```python
from build123d import *

# Parameters (mm, degrees)
ESBO_O1_R                = 2.975
RESSALTO_EXTRUS_O1_DEPTH = 10
ESBO_O2_R                = 4.073112834
ESBO_O2_R_2              = 2.425
CORTE_EXTRUS_O1_DEPTH    = 1.12
ESBO_O3_R                = 1.455
CORTE_EXTRUS_O2_DEPTH    = 1
ESBO_O4_R                = 1.975
CORTE_EXTRUS_O3_DEPTH    = 9
RESSALTO_EXTRUS_O2_START = 0.5
ESBO_O5_R                = 1.975
RESSALTO_EXTRUS_O2_DEPTH = 0.5
CHANFRO1_SIZE            = 0.25
ESBO_O6_W                = 0.8
ESBO_O6_H                = 6.683609012
CORTE_EXTRUS_O4_DEPTH    = 3
CHANFRO2_SIZE            = 0.5
ESBO_O7_W                = 0.7
ESBO_O7_H                = 5.908680056
RESSALTO_EXTRUS_O3_DEPTH = 6


with BuildPart() as part:
    # Esboço1 → Ressalto-extrusão1 (new body)
    with BuildSketch(Plane.XY):
        Circle(ESBO_O1_R)
    extrude(amount=RESSALTO_EXTRUS_O1_DEPTH)

    # Esboço2 → Corte-extrusão1 (cut)
    with BuildSketch(Plane(origin=(0, 0, 5.5), x_dir=(-1, 0, 0), z_dir=(0, 0, -1))):
        Circle(ESBO_O2_R)
        Circle(ESBO_O2_R_2, mode=Mode.SUBTRACT)
    extrude(amount=-CORTE_EXTRUS_O1_DEPTH, mode=Mode.SUBTRACT)

    # Esboço3 → Corte-extrusão2 (cut)
    with BuildSketch(Plane(origin=(0, 0, 0), x_dir=(-1, 0, 0), z_dir=(0, 0, -1))):
        Circle(ESBO_O3_R)
    extrude(amount=-CORTE_EXTRUS_O2_DEPTH, mode=Mode.SUBTRACT)

    # Esboço4 → Corte-extrusão3 (cut)
    with BuildSketch(Plane.XY.offset(10)):
        Circle(ESBO_O4_R)
    extrude(amount=-CORTE_EXTRUS_O3_DEPTH, mode=Mode.SUBTRACT)

    # Esboço5 → Ressalto-extrusão2 (add)
    with BuildSketch(Plane.XY.offset(1).offset(RESSALTO_EXTRUS_O2_START)):
        Circle(ESBO_O5_R)
    extrude(amount=-RESSALTO_EXTRUS_O2_DEPTH)

    # Chanfro1
    chanfro1_edges = [part.edges().sort_by_distance(p)[0] for p in [
        (-2.975, 0, 0),
        (-2.975, 0, 10),
    ]]
    chamfer(chanfro1_edges, length=CHANFRO1_SIZE)

    # Esboço6 → Corte-extrusão4 (cut)
    with BuildSketch(Plane.XY.offset(10)):
        Rectangle(ESBO_O6_W, ESBO_O6_H)
    extrude(amount=-CORTE_EXTRUS_O4_DEPTH, mode=Mode.SUBTRACT)

    # Chanfro2
    # the kernel refuses this chamfer: 0.5 mm, written as the material it takes off along each edge
    with BuildSketch(Plane(origin=(0.4, 0.64822805, 10), x_dir=(-0.027495876610586403, 0, -0.9996219169112968), z_dir=(0, 1, 0))) as chanfro2_piece_1:
        Polygon((CHANFRO2_SIZE * 0.999621916911, -CHANFRO2_SIZE * 0.0274958766106), (-CHANFRO2_SIZE * 0.0274958766106, -CHANFRO2_SIZE * 0.999621916911), (0, 0), align=None)
    extrude(amount=3.333095776, mode=Mode.SUBTRACT)
    with BuildSketch(Plane(origin=(0.4, -3.981323826, 10), x_dir=(0.9996219169112968, 0, 0.027495876610585633), z_dir=(0, 1, 0)), Plane(origin=(-0.4, -0.64822805, 10), x_dir=(-0.9996219169112968, 0, 0.027495876610585623), z_dir=(0, -1, 0)), Plane(origin=(-0.4, 3.981323826, 10), x_dir=(-0.9996219169112968, 0, 0.027495876610585623), z_dir=(0, -1, 0))) as chanfro2_piece_2:
        Polygon((CHANFRO2_SIZE * 0.999621916911, CHANFRO2_SIZE * 0.0274958766106), (-CHANFRO2_SIZE * 0.0274958766106, CHANFRO2_SIZE * 0.999621916911), (0, 0), align=None)
    extrude(amount=3.333095776, mode=Mode.SUBTRACT)

    # Esboço7 → Ressalto-extrusão3 (add)
    with BuildSketch(Plane.XY.offset(7)):
        Rectangle(ESBO_O7_W, ESBO_O7_H)
    extrude(amount=RESSALTO_EXTRUS_O3_DEPTH)


solid = part.part
```
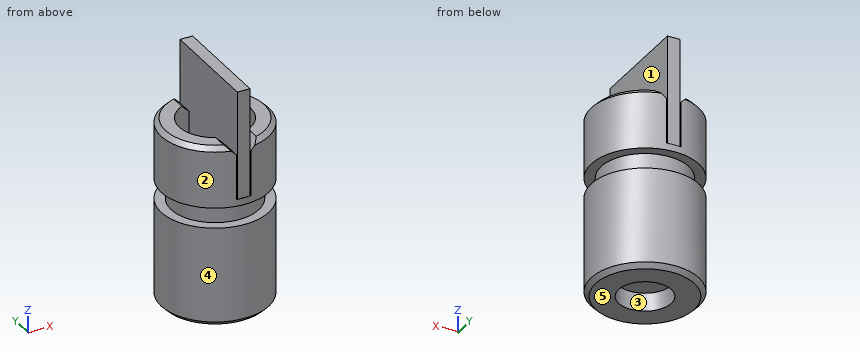
For this review, take the finished solid that the model builds, in its own axes (mm). Face numbers are marked on the shaded views. A direction names the side the tool comes from. Coordinates: 2 decimals unless noted, no trailing zeros. Loops run counter-clockwise (first coordinate to the right, second up) from the corner with the lowest first, then second, coordinate; pieces in that order, holes last. Notation, with made-up numbers: (87, 78.5) - (136, 78.5) arc R17 cw to (136, 103.5) - close; hole circle Ø4 at (-33, 8.25). An arc over 180 degrees is marked (long way). Use one line per item in the form item = value. Start each with the question number.
1) Take a section at B-B (x = 0). State the section outline as (y, z) points (3 decimals).
2) Draft analysis for pull direction X (two halves, no side actions). For the marked faces 3, 4 and 5, state which applies: released by +X, released by -X, zero draft, split by the parting line, or undercut.
3) Take a section at C-C (z = 4.25). State the section outline as (x, y) points (3 decimals), plus the area to 3 significant figures.
4) Take a section at A-A (y = 0). State the section outline as (x, z) points (3 decimals), plus the area to 3 significant figures.
5) For pin 1 (0.6 mm diameter, centred on x = 0, z = 9.5, fed in from +Y); pin 2 (1 mm diameter, centred on x = -0.5, z = 4.5, fed in from -Y) (3 decimals); pin 3 (0.8 mm diameter, centred on y = -2.5, z = 8, fed in from -X); pin 4 (1.5 mm diameter, centred on x = -1.5, y = -0.5, fed in from +Z), all flat-tipped, find the tip position at first contact; note any pin that passes through.
6) For the marked faces 1 and 2, list the 3-axis set-ups (+Z, -Z, +X, -X, +Y, -Y) from which the entire face can be reached by the end or side of a thin tool; tool diameter is ignored.
7) To check wall thickness, follow probe 1 along Z at (x, y) = (0.15, -0.45); probe 2 along Z at (x, y) = (1.2, 2.25); probe 3 along X at (y, z) = (0, 3.5) (3 decimals). State the ranges of each line that lie inside material, in increasing order. Write a range as from..to.
8) Take a section at D-D (z = 11). State the section outline as (x, y) points.
From the geometry:
q1.outline = (-2.975, 0.25) - (-2.725, 0) - (-1.455, 0) - (-1.455, 1) - (1.455, 1) - (1.455, 0) - (2.725, 0) - (2.975, 0.25) - (2.975, 5.5) - (2.425, 5.5) - (2.425, 6.62) - (2.975, 6.62) - (2.975, 7) - (2.954, 7) - (2.954, 13) - (-2.954, 13) - (-2.954, 7) - (-2.975, 7) - (-2.975, 6.62) - (-2.425, 6.62) - (-2.425, 5.5) - (-2.975, 5.5) - close; hole (-1.975, 1.5) - (1.975, 1.5) - (1.975, 7) - (-1.975, 7) - close
q2.face_3 = undercut
q2.face_4 = split by the parting line
q2.face_5 = zero draft
q3.outline = circle Ø5.95 at (0, 0); hole circle Ø3.95 at (0, 0)
q3.area = 15.6 mm2
q4.outline = (-2.975, 0.25) - (-2.725, 0) - (-1.455, 0) - (-1.455, 1) - (1.455, 1) - (1.455, 0) - (2.725, 0) - (2.975, 0.25) - (2.975, 5.5) - (2.425, 5.5) - (2.425, 6.62) - (2.975, 6.62) - (2.975, 9.75) - (2.725, 10) - (1.975, 10) - (1.975, 1.5) - (-1.975, 1.5) - (-1.975, 10) - (-2.725, 10) - (-2.975, 9.75) - (-2.975, 6.62) - (-2.425, 6.62) - (-2.425, 5.5) - (-2.975, 5.5) - close; (-0.35, 7) - (0.35, 7) - (0.35, 13) - (-0.35, 13) - close
q4.area = 25.9 mm2
q5.pin_1 = 2.95
q5.pin_2 = -2.975
q5.pin_3 = -2.11
q5.pin_4 = 10
q6.face_1 = +Z, +Y, -Y
q6.face_2 = +Z, -Z
q7.probe_1 = 1..1.5, 7..13
q7.probe_2 = 0..5.5, 6.62..10
q7.probe_3 = -2.975..-1.975, 1.975..2.975
q8.outline = (-0.35, -2.95) - (0.35, -2.95) - (0.35, 2.95) - (-0.35, 2.95) - close
